Could you check a few things on this model? Use its own coordinates, in mm. A direction names the side the tool comes from. Round coordinates to 2 decimals unless told otherwise and drop trailing zeros. Write each loop counter-clockwise with the first axis right and the second up, starting at its lowest first coordinate (ties: lowest second). Pieces come first, ordered by that corner, then holes. Notation, with made-up numbers: (21.25, 85.25) - (26.25, 85.25) arc R26 ccw to (26.25, 104.25) - close; hole circle Ø7 at (82, -31.75). An arc over 180 degrees is marked (long way). Put each result on its own line as item: value.
from build123d import *

# Parameters (mm, degrees)
ESQUISSE1_W                   = 44.2
ESQUISSE1_H                   = 52.2
BOSS_EXTRU_1_DEPTH            = 52.2
ENL_V_MAT_EXTRU_2_DEPTH       = 74.209903702
ENL_V_MAT_EXTRU_2_DEPTH_BACK  = 44.2
ENL_V_MAT_EXTRU_3_DEPTH       = 74.209903702
ENL_V_MAT_EXTRU_3_DEPTH_BACK  = 44.2
ENL_V_MAT_EXTRU_4_DEPTH       = 78.059003368
ENL_V_MAT_EXTRU_4_DEPTH_BACK  = 46
ENL_V_MAT_EXTRU_5_DEPTH       = 78.059003368
ENL_V_MAT_EXTRU_5_DEPTH_BACK  = 46
ENL_V_MAT_EXTRU_7_DEPTH       = 45.550224466
ENL_V_MAT_EXTRU_7_DEPTH_BACK  = 45.550224466
ENL_V_MAT_EXTRU_8_DEPTH       = 78.059003368
ENL_V_MAT_EXTRU_8_DEPTH_BACK  = 46
ENL_V_MAT_EXTRU_9_DEPTH       = 75.993733072
ENL_V_MAT_EXTRU_9_DEPTH_BACK  = 46
ESQUISSE13_W                  = 35
ESQUISSE13_H                  = 43
ENL_V_MAT_EXTRU_10_DEPTH      = 44
ENL_V_MAT_EXTRU_11_DEPTH      = 72.032809321
ENL_V_MAT_EXTRU_11_DEPTH_BACK = 1.5


with BuildPart() as part:
    # Esquisse1 → Boss.-Extru.1 (new body)
    with BuildSketch(Plane.XY):
        Rectangle(ESQUISSE1_W, ESQUISSE1_H)
    extrude(amount=BOSS_EXTRU_1_DEPTH)

    # Esquisse2 → Enlèv. mat.-Extru.2 (cut, two sides: drawn at the far end of the back side and taken through both)
    with BuildSketch(Plane(origin=(22.1, 0, 0), x_dir=(0, 0, -1), z_dir=(1, 0, 0)).offset(-ENL_V_MAT_EXTRU_2_DEPTH_BACK)):
        Polygon((-201.352290675, -19.9), (-52.2, -19.9), (-28.55, -19.9), (-28.55, -21.45), (-32.25, -21.45), (-32.25, -22.45), (-28.745559959, -26.1), (74.553898465, -133.690091099), (-39.180744024, -409.461834307), (-315.086933163, -295.671743208), align=None)
    extrude(amount=ENL_V_MAT_EXTRU_2_DEPTH + ENL_V_MAT_EXTRU_2_DEPTH_BACK, mode=Mode.SUBTRACT)

    # Esquisse3 → Enlèv. mat.-Extru.3 (cut, two sides: drawn at the far end of the back side and taken through both)
    with BuildSketch(Plane(origin=(22.1, 0, 0), x_dir=(0, 0, -1), z_dir=(1, 0, 0)).offset(-ENL_V_MAT_EXTRU_3_DEPTH_BACK)):
        Polygon((149.152290675, -19.9), (0, -19.9), (-23.65, -19.9), (-23.65, -21.45), (-19.95, -21.45), (-19.95, -22.45), (-23.454440041, -26.1), (-126.753898465, -133.690091099), (-13.019255976, -409.461834307), (262.886933163, -295.671743208), align=None)
    extrude(amount=ENL_V_MAT_EXTRU_3_DEPTH + ENL_V_MAT_EXTRU_3_DEPTH_BACK, mode=Mode.SUBTRACT)

    # Esquisse4 → Enlèv. mat.-Extru.4 (cut, two sides: drawn at the far end of the back side and taken through both)
    with BuildSketch(Plane(origin=(0, 26.1, 0), x_dir=(1, 0, 0), z_dir=(0, 1, 0)).offset(-ENL_V_MAT_EXTRU_4_DEPTH_BACK)):
        Polygon((-15.9, -191.333109619), (-15.9, -52.2), (-15.9, -28.55), (-17.45, -28.55), (-17.45, -32.25), (-18.45, -32.25), (-22.1, -28.745559959), (-122.462816227, 67.614843274), (-379.791464965, -38.281593439), (-273.228648738, -297.229546332), align=None)
    extrude(amount=ENL_V_MAT_EXTRU_4_DEPTH + ENL_V_MAT_EXTRU_4_DEPTH_BACK, mode=Mode.SUBTRACT)

    # Esquisse5 → Enlèv. mat.-Extru.5 (cut, two sides: drawn at the far end of the back side and taken through both)
    with BuildSketch(Plane(origin=(0, 26.1, 0), x_dir=(1, 0, 0), z_dir=(0, 1, 0)).offset(-ENL_V_MAT_EXTRU_5_DEPTH_BACK)):
        Polygon((-15.9, 139.133109619), (-15.9, 0), (-15.9, -23.65), (-17.45, -23.65), (-17.45, -19.95), (-18.45, -19.95), (-22.1, -23.454440041), (-122.462816228, -119.814843274), (-379.791464965, -13.918406561), (-273.228648738, 245.029546332), align=None)
    extrude(amount=ENL_V_MAT_EXTRU_5_DEPTH + ENL_V_MAT_EXTRU_5_DEPTH_BACK, mode=Mode.SUBTRACT)

    # Esquisse6 → Enlèv. mat.-Extru.7 (cut, two sides: drawn at the far end of the back side and taken through both)
    with BuildSketch(Plane.XY.offset(28.55).offset(-ENL_V_MAT_EXTRU_7_DEPTH_BACK)):
        Polygon((-161.22284167, -19.9), (-22.1, -19.9), (-15.9, -19.9), (-15.9, -26.093649616), (-15.9, -165.216491285), (-212.645110561, -361.97019968), (-357.967952231, -216.653708395), align=None)
    extrude(amount=ENL_V_MAT_EXTRU_7_DEPTH + ENL_V_MAT_EXTRU_7_DEPTH_BACK, mode=Mode.SUBTRACT)

    # Esquisse11 → Enlèv. mat.-Extru.8 (cut, two sides: drawn at the far end of the back side and taken through both)
    with BuildSketch(Plane(origin=(0, 26.1, 0), x_dir=(1, 0, 0), z_dir=(0, 1, 0)).offset(-ENL_V_MAT_EXTRU_8_DEPTH_BACK)):
        Polygon((164.227968273, -49.1), (22.1, -49.1), (-15.9, -49.1), (-158.027968273, -49.1), (-158.027968273, -333.355936546), (164.227968273, -333.355936546), align=None)
    extrude(amount=ENL_V_MAT_EXTRU_8_DEPTH + ENL_V_MAT_EXTRU_8_DEPTH_BACK, mode=Mode.SUBTRACT)

    # Esquisse12 → Enlèv. mat.-Extru.9 (cut, two sides: drawn at the far end of the back side and taken through both)
    with BuildSketch(Plane(origin=(0, 26.1, 0), x_dir=(1, 0, 0), z_dir=(0, 1, 0)).offset(-ENL_V_MAT_EXTRU_9_DEPTH_BACK)):
        Polygon((159.687460199, -3.1), (22.1, -3.1), (-15.9, -3.1), (-153.487460199, -3.1), (-153.487460199, 272.074920398), (159.687460199, 272.074920398), align=None)
    extrude(amount=ENL_V_MAT_EXTRU_9_DEPTH + ENL_V_MAT_EXTRU_9_DEPTH_BACK, mode=Mode.SUBTRACT)

    # Esquisse13 → Enlèv. mat.-Extru.10 (cut)
    with BuildSketch(Plane(origin=(0, 26.1, 0), x_dir=(1, 0, 0), z_dir=(0, 1, 0))):
        with Locations((3.1, -26.1)):
            Rectangle(ESQUISSE13_W, ESQUISSE13_H)
    extrude(amount=-ENL_V_MAT_EXTRU_10_DEPTH, mode=Mode.SUBTRACT)

    # Esquisse14 → Enlèv. mat.-Extru.11 (cut, two sides: drawn at the far end of the back side and taken through both)
    with BuildSketch(Plane(origin=(22.1, 0, 0), x_dir=(0, 0, -1), z_dir=(1, 0, 0)).offset(-ENL_V_MAT_EXTRU_11_DEPTH_BACK)):
        with BuildLine():
            Line((-21.6, 4.6), (-21.6, 26.1))
            Line((-21.6, 26.1), (-30.6, 26.1))
            Line((-30.6, 26.1), (-30.6, 4.6))
            ThreePointArc((-30.6, 4.6), (-26.1, 0.1), (-21.6, 4.6))
        make_face()
    extrude(amount=ENL_V_MAT_EXTRU_11_DEPTH + ENL_V_MAT_EXTRU_11_DEPTH_BACK, mode=Mode.SUBTRACT)


solid = part.part
(1) Imagine slicing it at D-D, the plane x = -5. List the corners of the cut face in (y, z) for me.
Values found:
outline: (-26.1, 23.45) - (-22.45, 19.95) - (-21.45, 19.95) - (-21.45, 23.65) - (-19.9, 23.65) - (-19.9, 3.1) - (26.1, 3.1) - (26.1, 4.6) - (-17.9, 4.6) - (-17.9, 47.6) - (26.1, 47.6) - (26.1, 49.1) - (-19.9, 49.1) - (-19.9, 28.55) - (-21.45, 28.55) - (-21.45, 32.25) - (-22.45, 32.25) - (-26.1, 28.75) - close
(2) For faces 4 (the face through (21.3, 0.1, 26.2)), 5 (the face through (-17, 3, 23.65)), 6 (the face through (-17.45, 3, 30)), 7 (the face through (20.6, -0.5, 26.4)), which set-ups out of +Z, -Z, +X, -X, +Y, -Y let a thin tool reach every point of the face, with its end or its side?
Values found:
face 4: +X, +Y
face 5: -Z, +Y, -Y
face 6: +Z, +Y, -Y
face 7: +Y
(3) I'm going to push flat-ended pins straight in: pin 1 (1 mm diameter, centred on x = 8, z = 18.5, fed in from +Y); pin 2 (3 mm diameter, centred on y = -24, z = 28, fed in from -X); pin 3 (0.8 mm diameter, centred on x = 3, y = -22, fed in from +Z); pin 4 (4 mm diameter, centred on y = 6.5, z = 22.5, fed in from -X). Where does each tip first touch, or does it pass through?
Values found:
pin 1: stops at y = -17.9
pin 2: stops at x = -15.9
pin 3: stops at z = 32.25
pin 4: stops at x = -22.1
(4) Imagine slicing it at B-B, the plane z = 26.1. List the corners of the cut face in (x, y) for me, then the cut area to 3 significant figures.
Values found:
outline: (-22.1, -19.9) - (-15.9, -19.9) - (-15.9, -26.1) - (22.1, -26.1) - (22.1, 0.1) - (20.6, 0.1) - (20.6, -17.9) - (-14.4, -17.9) - (-14.4, 26.1) - (-22.1, 26.1) - close
area: 690 mm^2
(5) If we mould it in two halves opening along Y, with no side actions, what happens to faces 1 (the face through (3, -17.9, 26)), 2 (the face through (3, -26.1, 26)), 3 (the face through (3, -21.45, 30))? For each: pulls with the +Y half, pulls with the -Y half, needs draft (parallel to the pull), parting line crosses it, or undercut.
Values found:
face 1: pulls with the +Y half
face 2: pulls with the -Y half
face 3: undercut
(6) Please list where these lines run through material, in increasing order: probe 1 along X at (y, z) = (-7, 38); probe 2 along Z at (x, y) = (-8, 10); probe 3 along Y at (x, z) = (-2, 41.5). Write a range as from..to.
Values found:
probe 1: x = -15.9..-14.4, 20.6..22.1
probe 2: z = 3.1..4.6, 47.6..49.1
probe 3: y = -19.9..-17.9
(7) Imagine slicing it at A-A, the plane y = -13. List the corners of the cut face in (x, z) for me, then the cut area to 3 significant figures.
Values found:
outline: (-22.1, 23.45) - (-18.45, 19.95) - (-17.45, 19.95) - (-17.45, 23.65) - (-15.9, 23.65) - (-15.9, 3.1) - (22.1, 3.1) - (22.1, 49.1) - (-15.9, 49.1) - (-15.9, 28.55) - (-17.45, 28.55) - (-17.45, 32.25) - (-18.45, 32.25) - (-22.1, 28.75) - close; hole (-14.4, 4.6) - (20.6, 4.6) - (20.6, 47.6) - (-14.4, 47.6) - close
area: 295 mm^2
(8) Imagine slicing it at C-C, the plane y = 8.5. List the corners of the cut face in (x, z) for me, then the cut area to 3 significant figures.
Values found:
outline: (-22.1, 23.45) - (-18.45, 19.95) - (-17.45, 19.95) - (-17.45, 23.65) - (-15.9, 23.65) - (-15.9, 3.1) - (22.1, 3.1) - (22.1, 21.6) - (20.6, 21.6) - (20.6, 4.6) - (-14.4, 4.6) - (-14.4, 47.6) - (20.6, 47.6) - (20.6, 30.6) - (22.1, 30.6) - (22.1, 49.1) - (-15.9, 49.1) - (-15.9, 28.55) - (-17.45, 28.55) - (-17.45, 32.25) - (-18.45, 32.25) - (-22.1, 28.75) - close
area: 281 mm^2
